Geometry check sheet. Reference: the model listing, model coordinates, mm. A direction names the side the tool comes from. Round coordinates to 2 decimals unless told otherwise and drop trailing zeros. Loops run counter-clockwise (first coordinate to the right, second up) from the corner with the lowest first, then second, coordinate; pieces in that order, holes last. Notation, with made-up numbers: M -4,86.25 L 21,86.25 A20 cw 21,119.25 Z; hole C 59,-34 d6. An arc over 180 degrees is marked long. Use one line per item in the form item = value. Start each with the question number.
1. Draft check along Y on faces 4 (the flat face through (-102, 11, -61)), 5 (the flat face through (-10, 7.5, -22.7)), 6 (the cylindrical face through (-102.535, 9.676, -53.254)). Enter one of: pulls with the +Y half, pulls with the -Y half, needs draft (parallel to the pull), parting line crosses it, or undercut.
2. Set-up check for faces 1 (the flat face through (-5, 7, -95)), 2 (the cylindrical face through (-4.93, 7.509, -23.056)), 3 (the flat face through (-98, 4, -77)): record each of +Z, -Z, +X, -X, +Y, -Y from which the full face is reachable in a straight line by a thin tool's end or side.
3. Cross-section at B-B (z = -12.5). Record the boundary of the cut face in (x, y).
4. Cross-section at C-C (x = -5). Record the boundary of the cut face in (y, z).
5. Cross-section at D-D (z = -83). Record the boundary of the cut face in (x, y).
6. Material ranges on line 1 (Z direction, x = -74.5, y = 11); line 2 (X direction, y = 8.75, z = -17); line 3 (Z direction, x = -44.5, y = 7.75), recorded low to high.
7. Cross-section at A-A (y = 13). State how many separate pieces and enclosed holes the cut face has, then the cut area to 3 significant figures.
8. Go/stop test with flat-tipped pins: pin 1 (8 mm diameter, centred on x = -83.5, z = -67, fed in from +Y); pin 2 (6.5 mm diameter, centred on x = -48.5, z = -93.5, fed in from -Y). Record where each tip stops, or that it passes through.
```python
from build123d import *

# Parameters (mm, degrees)
SKETCH_1_W           = 105
SKETCH_1_H           = 100
EXTRUDE_1_DEPTH      = 16
CUT_EXTRUDE_5_REACH  = 147.88
SKETCH_8_R           = 1.45
CUT_EXTRUDE_7_DEPTH  = 146.880087743
SKETCH_9_W           = 35
SKETCH_9_H           = 16
EXTRUDE_2_DEPTH      = 5
SKETCH_10_R          = 2.25
CUT_EXTRUDE_8_DEPTH  = 5
SKETCH_12_W          = 20
SKETCH_12_H          = 16
EXTRUDE_3_DEPTH      = 10
SKETCH_13_R          = 2.25
CUT_EXTRUDE_10_DEPTH = 5
SKETCH_14_W          = 105
SKETCH_14_H          = 100
CUT_EXTRUDE_11_DEPTH = 2
SKETCH_15_R          = 1.5
CUT_EXTRUDE_12_DEPTH = 4
SKETCH_16_W          = 85
SKETCH_16_H          = 25
CUT_EXTRUDE_13_DEPTH = 3
CHAMFER_1_SIZE       = 3
SKETCH_17_R          = 2.25
CUT_EXTRUDE_14_DEPTH = 5
SKETCH_18_R          = 1.5
CUT_EXTRUDE_15_DEPTH = 4
SKETCH_21_R          = 2.45
CUT_EXTRUDE_17_DEPTH = 13.2


with BuildPart() as part:
    # 草图1 → 凸台-拉伸1 (new body)
    with BuildSketch(Plane(origin=(0, 0, 0), x_dir=(1, 0, 0), z_dir=(0, 1, 0))):
        with Locations((-52.5, 50)):
            Rectangle(SKETCH_1_W, SKETCH_1_H)
    extrude(amount=EXTRUDE_1_DEPTH)

    # 草图6 → 切除-拉伸5 (cut, up to next)
    with BuildSketch(Plane(origin=(0, 16, 0), x_dir=(1, 0, 0), z_dir=(0, 1, 0)), mode=Mode.PRIVATE) as cut_extrude_5_sk1:
        Polygon((-45.224064051, 40), (-5, 40), (-5, 5), (-70, 5), (-70, 20), (-100, 20), (-100, 40), align=None)
    cut_extrude_5_tool1 = extrude(cut_extrude_5_sk1.sketch, amount=-CUT_EXTRUDE_5_REACH, mode=Mode.PRIVATE) & part.part
    # 草图6 → 切除-拉伸5 (cut, up to next)
    with BuildSketch(Plane(origin=(0, 16, 0), x_dir=(1, 0, 0), z_dir=(0, 1, 0)), mode=Mode.PRIVATE) as cut_extrude_5_sk2:
        Polygon((-70, 95), (-5, 95), (-5, 60), (-45.224064051, 60), (-100, 60), (-100, 80), (-70, 80), align=None)
    cut_extrude_5_tool2 = extrude(cut_extrude_5_sk2.sketch, amount=-CUT_EXTRUDE_5_REACH, mode=Mode.PRIVATE) & part.part
    add(cut_extrude_5_tool1.solids().sort_by_distance((-47.413043, 16, -24.065217))[0], mode=Mode.SUBTRACT)
    add(cut_extrude_5_tool2.solids().sort_by_distance((-47.413043, 16, -75.934783))[0], mode=Mode.SUBTRACT)

    # 草图8 → 切除-拉伸7 (cut, through all)
    with BuildSketch(Plane(origin=(0, 16, 0), x_dir=(1, 0, 0), z_dir=(0, 1, 0))):
        with Locations(Location((-102, 97, 0), (0, 0, 270))):
            Circle(SKETCH_8_R)
        with Locations(Location((-102, 83, 0), (0, 0, 270))):
            Circle(SKETCH_8_R)
        with Locations(Location((-78, 97, 0), (0, 0, 270))):
            Circle(SKETCH_8_R)
        with Locations(Location((-78, 83, 0), (0, 0, 270))):
            Circle(SKETCH_8_R)
        with Locations(Location((-78, 17, 0), (0, 0, 90))):
            Circle(SKETCH_8_R)
        with Locations(Location((-78, 3, 0), (0, 0, 90))):
            Circle(SKETCH_8_R)
        with Locations(Location((-102, 17, 0), (0, 0, 90))):
            Circle(SKETCH_8_R)
        with Locations(Location((-102, 3, 0), (0, 0, 90))):
            Circle(SKETCH_8_R)
    extrude(amount=-CUT_EXTRUDE_7_DEPTH, mode=Mode.SUBTRACT)

    # 草图9 → 凸台-拉伸2 (add)
    with BuildSketch(Plane.ZY.offset(5)):
        with Locations((-22.5, 8)):
            Rectangle(SKETCH_9_W, SKETCH_9_H)
        with Locations((-77.5, 8)):
            Rectangle(SKETCH_9_W, SKETCH_9_H)
    extrude(amount=EXTRUDE_2_DEPTH)

    # 草图10 → 切除-拉伸8 (cut)
    with BuildSketch(Plane(origin=(0, 16, 0), x_dir=(1, 0, 0), z_dir=(0, 1, 0))):
        with Locations(Location((-5, 95, 0), (0, 0, 270))):
            Circle(SKETCH_10_R)
        with Locations(Location((-5, 5, 0), (0, 0, 90))):
            Circle(SKETCH_10_R)
    extrude(amount=-CUT_EXTRUDE_8_DEPTH, mode=Mode.SUBTRACT)

    # 草图12 → 凸台-拉伸3 (add)
    with BuildSketch(Plane(origin=(-100, 0, 0), x_dir=(0, 0, -1), z_dir=(1, 0, 0))):
        with Locations((30, 8)):
            Rectangle(SKETCH_12_W, SKETCH_12_H)
        with Locations((70, 8)):
            Rectangle(SKETCH_12_W, SKETCH_12_H)
    extrude(amount=EXTRUDE_3_DEPTH)

    # 草图13 → 切除-拉伸10 (cut)
    with BuildSketch(Plane(origin=(0, 16, 0), x_dir=(1, 0, 0), z_dir=(0, 1, 0))):
        with Locations(Location((-100.5, 50, 0), (0, 0, 270))):
            Circle(SKETCH_13_R)
        with Locations(Location((-100.5, 60, 0), (0, 0, 270))):
            Circle(SKETCH_13_R)
    extrude(amount=-CUT_EXTRUDE_10_DEPTH, mode=Mode.SUBTRACT)

    # 草图14 → 切除-拉伸11 (cut)
    with BuildSketch(Plane.XZ):
        with Locations((-52.5, -50)):
            Rectangle(SKETCH_14_W, SKETCH_14_H)
    extrude(amount=-CUT_EXTRUDE_11_DEPTH, mode=Mode.SUBTRACT)

    # 草图15 → 切除-拉伸12 (cut)
    with BuildSketch(Plane(origin=(0, 11, 0), x_dir=(1, 0, 0), z_dir=(0, 1, 0))):
        with Locations(Location((-5, 5, 0), (0, 0, 270))):
            Circle(SKETCH_15_R)
        with Locations(Location((-5, 95, 0), (0, 0, 270))):
            Circle(SKETCH_15_R)
        with Locations(Location((-100.5, 60, 0), (0, 0, 270))):
            Circle(SKETCH_15_R)
        with Locations(Location((-100.5, 50, 0), (0, 0, 270))):
            Circle(SKETCH_15_R)
    extrude(amount=-CUT_EXTRUDE_12_DEPTH, mode=Mode.SUBTRACT)

    # 草图16 → 切除-拉伸13 (cut)
    with BuildSketch(Plane.XZ.offset(-2)):
        with Locations((-62.5, -12.5)):
            Rectangle(SKETCH_16_W, SKETCH_16_H)
        with Locations((-62.5, -87.5)):
            Rectangle(SKETCH_16_W, SKETCH_16_H)
    extrude(amount=-CUT_EXTRUDE_13_DEPTH, mode=Mode.SUBTRACT)

    # 倒角1
    chamfer_1_edges = [part.edges().sort_by_distance(p)[0] for p in [
        (-20, 5, -2.5),
        (-97.5, 5, -25),
        (-97.5, 5, -75),
        (-20, 5, -97.5),
    ]]
    chamfer(chamfer_1_edges, length=CHAMFER_1_SIZE - 0.0001)  # a hair under: the kernel refuses the full size

    # 草图17 → 切除-拉伸14 (cut)
    with BuildSketch(Plane.ZY.offset(105)):
        with Locations((-55.4, 9)):
            Circle(SKETCH_17_R)
    extrude(amount=-CUT_EXTRUDE_14_DEPTH, mode=Mode.SUBTRACT)

    # 草图18 → 切除-拉伸15 (cut)
    with BuildSketch(Plane.ZY.offset(100)):
        with Locations((-55.4, 9)):
            Circle(SKETCH_18_R)
    extrude(amount=-CUT_EXTRUDE_15_DEPTH, mode=Mode.SUBTRACT)

    # 草图21 → 切除-拉伸17 (cut)
    with BuildSketch(Plane(origin=(0, 0, 0), x_dir=(0, 0, -1), z_dir=(1, 0, 0))):
        with Locations((25, 9)):
            Circle(SKETCH_21_R)
        with Locations((75, 9)):
            Circle(SKETCH_21_R)
    extrude(amount=-CUT_EXTRUDE_17_DEPTH, mode=Mode.SUBTRACT)


solid = part.part
```
Reported:
q1.face_4 = pulls with the +Y half
q1.face_5 = needs draft
q1.face_6 = undercut
q2.face_1 = +Y
q2.face_2 = +X
q2.face_3 = -Z, -X, -Y
q3.outline = M -105,5 L -70,5 L -70,16 L -105,16 Z; M -10,2 L 0,2 L 0,16 L -10,16 Z
q4.outline = M 2,-100 L 16,-100 L 16,-97.25 L 11,-97.25 L 11,-96.5 L 7,-96.5 L 7,-93.5 L 11,-93.5 L 11,-92.75 L 16,-92.75 L 16,-7.25 L 11,-7.25 L 11,-6.5 L 7,-6.5 L 7,-3.5 L 11,-3.5 L 11,-2.75 L 16,-2.75 L 16,0 L 2,0 Z; hole C 9,-75 d4.9; hole C 9,-25 d4.9
q5.outline = M -105,5 L -103.45,5 L -103.45,16 L -105,16 Z; M -100.55,5 L -79.45,5 L -79.45,16 L -100.55,16 Z; M -76.55,5 L -70,5 L -70,16 L -76.55,16 Z; M -10,2 L 0,2 L 0,16 L -10,16 Z
q6.line_1 = -100 to -80, -60 to -40, -20 to 0
q6.line_2 = -105 to -103.45, -100.55 to -79.45, -76.55 to -70, -10 to 0
q6.line_3 = -100 to -95, -60 to -40, -5 to 0
q7.separate_pieces = 1
q7.enclosed_holes = 14
q7.area = 5,380 mm²
q8.pin_1 = through
q8.pin_2 = 5
